Build history of the part. All positions in model axes, mm. A direction names the side the tool comes from. Give positions to 0.01 mm unless a question says otherwise; leave off trailing zeros. Order: outer loops, then holes, each group sorted by start corner. A loop starts at its lowest first (then second) coordinate and runs counter-clockwise, first axis right, second up. Notation, with made-up numbers: (-8, -7) - (14, -7) arc R5 cw to (14, 1) - close; hole circle Ø9 at (-27, -24). An arc over 180 degrees is marked (long way). Use a Markdown table: item, result. Add a question column.
(1) Mould opens along X. For faces 1 (the face through (3.5, -1, 6)), 2 (the face through (0, -6, 5)), 3 (the face through (0, 3, 4.7)), 4 (the face through (-3, 4.5, 2.5)) say: +X half, -X half, draft (parallel to the pull), parting line (faces both ways), or undercut.
(2) Slice it at D-D (z = 10.75). Write the cut outline in (x, y).
(3) Which spindle directions (+Z, -Z, +X, -X, +Y, -Y) get a long thin tool onto all of the face, cutting with end or side? Do faces 5 (the face through (4, -0.1, 2.5)), 6 (the face through (0, 4, 2)), 7 (the face through (-3.5, 6, 2.5)), 8 (the face through (-3.5, -2, 5)). Say none if no direction does.
(4) Slice it at A-A (y = -5.25). Write the cut outline in (x, z).
(5) Wall check: line 1 (Z direction, x = 0, y = 2.2); line 2 (Z direction, x = 0, y = 1.05); line 3 (Z direction, x = 0.75, y = 7.75). Give the ranges that are in metal, low to high.
(6) Slice it at B-B (x = 0). Write the cut outline in (y, z).
(7) Slice it at C-C (y = 4). Write the cut outline in (x, z), then the cut area to 3 significant figures.
(8) Flat gauge pins, fed straight in: pin 1 (4 mm diameter, centred on y = -1, z = 3.5, fed in from +X); pin 2 (2 mm diameter, centred on y = 2.5, z = 9.5, fed in from +X); pin 3 (0.8 mm diameter, centred on y = 5, z = 2.5, fed in from -X); pin 4 (3.5 mm diameter, centred on x = 1, z = 7.5, fed in from +Y). Where does each tip first touch, or does it go through?
from build123d import *

# Parameters (mm, degrees)
SKETCH_W          = 12
SKETCH_H          = 16
PAD_DEPTH         = 2
SKETCH001_R       = 2.5
PAD001_DEPTH      = 6
PAD001_DEPTH_BACK = 3
SKETCH002_R       = 2.95
POCKET_DEPTH      = 1
SKETCH003_W       = 1
SKETCH003_H       = 12
PAD002_DEPTH      = 1


with BuildPart() as part:
    # Sketch → Pad (new body)
    with BuildSketch(Plane.XY):
        Rectangle(SKETCH_W, SKETCH_H)
    extrude(amount=PAD_DEPTH)

    # Sketch001 → Pad001 (join, two sides)
    with BuildSketch(Plane.XZ) as pad001_sk:
        with BuildLine():
            Line((-3.5, 2), (-3.5, 8))
            ThreePointArc((3.5, 8), (0, 11.5), (-3.5, 8))
            Line((3.5, 8), (3.5, 2))
            Line((-3.5, 2), (3.5, 2))
        make_face()
        with Locations((0, 8)):
            Circle(SKETCH001_R, mode=Mode.SUBTRACT)
    extrude(amount=PAD001_DEPTH)
    extrude(pad001_sk.sketch, amount=-PAD001_DEPTH_BACK)

    # Sketch002 (on Face7 of Pad001) → Pocket (cut)
    with BuildSketch(Plane(origin=(0, 3, 0), x_dir=(-1, 0, 0), z_dir=(0, 1, 0))):
        with Locations((0, 8)):
            Circle(SKETCH002_R)
    extrude(amount=-POCKET_DEPTH, mode=Mode.SUBTRACT)

    # Sketch003 (on Face5 of Pocket) → Pad002 (join)
    with BuildSketch(Plane.XY.offset(2)):
        with Locations((-3.5, 0)):
            Rectangle(SKETCH003_W, SKETCH003_H)
        with Locations((3.5, 0)):
            Rectangle(SKETCH003_W, SKETCH003_H)
    extrude(amount=PAD002_DEPTH)


solid = part.part
Solution:
| question | item | result |
|---|---|---|
| 1 | face 1 | +X half |
| 1 | face 2 | draft |
| 1 | face 3 | undercut |
| 1 | face 4 | undercut |
| 2 | outline | (-2.17, -6) - (2.17, -6) - (2.17, 3) - (1.07, 3) - (1.07, 2) - (-1.07, 2) - (-1.07, 3) - (-2.17, 3) - close |
| 3 | face 5 | +Z, +X, +Y, -Y |
| 3 | face 6 | +Z |
| 3 | face 7 | +Z, +X, -X, +Y |
| 3 | face 8 | +Z, -X, +Y, -Y |
| 4 | outline | (-6, 0) - (6, 0) - (6, 2) - (4, 2) - (4, 3) - (3.5, 3) - (3.5, 8) arc R3.5 ccw to (-3.5, 8) - (-3.5, 3) - (-4, 3) - (-4, 2) - (-6, 2) - close; hole circle Ø5 at (0, 8) |
| 5 | line 1 | 0 to 5.05, 10.95 to 11.5 |
| 5 | line 2 | 0 to 5.5, 10.5 to 11.5 |
| 5 | line 3 | 0 to 2 |
| 6 | outline | (-8, 0) - (8, 0) - (8, 2) - (3, 2) - (3, 5.05) - (2, 5.05) - (2, 5.5) - (-6, 5.5) - (-6, 2) - (-8, 2) - close; (-6, 10.5) - (2, 10.5) - (2, 10.95) - (3, 10.95) - (3, 11.5) - (-6, 11.5) - close |
| 7 | outline | (-6, 0) - (6, 0) - (6, 2) - (4, 2) - (4, 3) - (3, 3) - (3, 2) - (-3, 2) - (-3, 3) - (-4, 3) - (-4, 2) - (-6, 2) - close |
| 7 | area | 26.0 mm2 |
| 8 | pin 1 | x = 6 |
| 8 | pin 2 | x = 3.46 |
| 8 | pin 3 | x = -4 |
| 8 | pin 4 | y = 2 |
